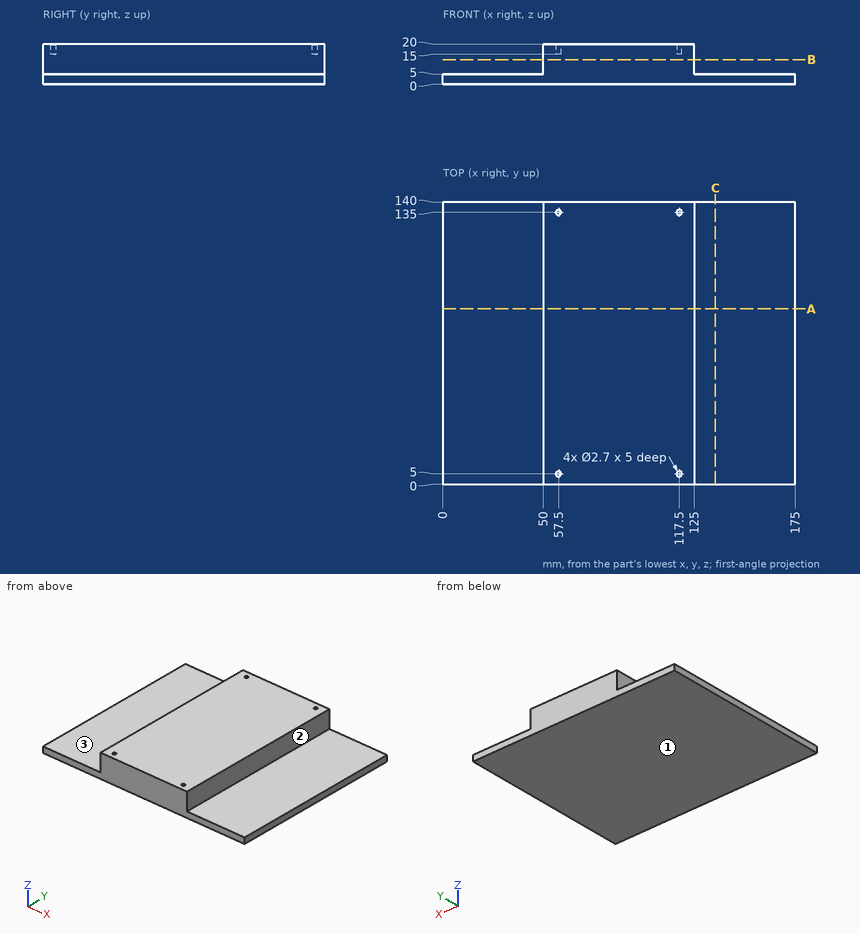
Answer from the drawing. Dimensions are ordinates in mm from the lowest x, y and z of the part. A direction names the side the tool comes from. Coordinates: 2 decimals unless noted, no trailing zeros. Order: outer loops, then holes, each group sorted by start corner. A loop starts at its lowest first (then second) coordinate and runs counter-clockwise, first axis right, second up. Notation, with made-up numbers: (-9, -30.75) - (37, -30.75) arc R21 ccw to (37, -8.75) - close; hole circle Ø2 at (-1.5, 39). An arc over 180 degrees is marked (long way). Use one line per item in the form item = value.
(1) Section B-B, the plane z = 12.25 is taken. Give the vertices of the cut face in (x, y), then the cut area to 3 significant figures.
Computed values:
outline = (50, 0) - (125, 0) - (125, 140) - (50, 140) - close
area = 10,500 mm²
(2) Section A-A, the plane y = 87 is taken. Give the vertices of the cut face in (x, z).
Computed values:
outline = (0, 0) - (175, 0) - (175, 5) - (125, 5) - (125, 20) - (50, 20) - (50, 5) - (0, 5) - close
(3) Straight lines are drawn through the part: L1, parallel to Y at x = 57.5, z = 16.45; L2, parallel to X at y = 135, z = 18.55; L3, parallel to Z at x = 153, y = 96. For each, find the intervals that lie inside material, in ascending order.
Computed values:
L1 = 0 to 3.65, 6.35 to 133.65, 136.35 to 140
L2 = 50 to 56.15, 58.85 to 116.15, 118.85 to 125
L3 = 0 to 5
(4) Which of the six approach directions +Z, -Z, +X, -X, +Y, -Y give full straight-line access (tool end or side, diameter ignored) to the marked faces 1, 2 and 3?
Computed values:
face_1 = -Z, +X, -X, +Y, -Y
face_2 = +Z, +X, +Y, -Y
face_3 = +Z, -X, +Y, -Y
(5) Section C-C, the plane x = 135.5 is taken. Give the vertices of the cut face in (y, z).
Computed values:
outline = (0, 0) - (140, 0) - (140, 5) - (0, 5) - close
(6) Given pin 1 Ø8 at (x, y) = (40.5, 49) entering from -Z; pin 2 Ø15 at (x, y) = (24.5, 64.5) entering from +Z; pin 3 Ø0.8 at (x, y) = (58, 5.5) entering from +Z; pin 4 Ø7.5 at (y, z) = (52, 12) entering from +X, each flat-ended and moving along its own axis, determine where each tip first touches the part or whether it passes through.
Computed values:
pin_1 = 0
pin_2 = 5
pin_3 = 15
pin_4 = 125
